Part model, mm, in its own coordinate system. A direction names the side the tool comes from. Give positions to 0.01 mm unless a question says otherwise; leave off trailing zeros. Order: outer loops, then holes, each group sorted by start corner. A loop starts at its lowest first (then second) coordinate and runs counter-clockwise, first axis right, second up. Notation, with made-up numbers: (-23.5, 15.5) - (15.5, 15.5) arc R25 ccw to (15.5, 32.5) - close; hole circle Ø2 at (-4.5, 84.25). An arc over 180 degrees is marked (long way). One line per item, written item: value.
```python
from build123d import *

# Parameters (mm, degrees)
F0_R     = 11.1125
F0_R_2   = 6.35
F1_DEPTH = 250.825
F2_DEPTH = 53.975
F3_SIZE2 = 1.5875
F3_SIZE  = 1.5875


with BuildPart() as f1:
    # F0 (on Top) → F1 (new body)
    with BuildSketch(Plane.XY):
        Circle(F0_R)
        Circle(F0_R_2, mode=Mode.SUBTRACT)
        Circle(F0_R_2)
    extrude(amount=F1_DEPTH)

    # F0 (on Top) → F2 (join)
    with BuildSketch(Plane.XY):
        Circle(F0_R_2)
    extrude(amount=-F2_DEPTH)

    # F3
    f3_edges = [f1.edges().sort_by_distance(p)[0] for p in [
        (-11.1125, 0, 250.825),
        (-6.35, 0, -53.975),
    ]]
    chamfer(f3_edges, length=F3_SIZE, length2=F3_SIZE2)


solid = f1.part
```
1) Wall check: line 1 along Z through (x, y) = (5.75, -4.75) (3 decimals); line 2 along Y through (x, z) = (-0.5, 16); line 3 along Y through (x, z) = (8.75, 136). Give the ranges that are in metal, low to high. Write a range as [from, to].
Answer:
line 1: z = [0, 250.825]
line 2: y = [-11.1, 11.1]
line 3: y = [-6.85, 6.85]
2) Slice it at C-C on z = 80.5. Write the cut outline in (x, y) (1 decimal), then the cut area to 3 significant figures.
Answer:
outline: circle Ø22.2 at (0, 0)
area: 388 mm2
3) Which spindle directions (+Z, -Z, +X, -X, +Y, -Y) get a long thin tool onto all of the face, cutting with end or side? Do faces 1 (the face through (-1.38, -6.2, -25.83)), 2 (the face through (0, 0, 250.825)). Say none if no direction does.
Answer:
face 1: -Z
face 2: +Z, +X, -X, +Y, -Y
4) Drop flat-ended pins along their axis: P1, Ø2, axis at x = 7.5, y = 0.5, coming from the -Z side; P2, Ø12, axis at x = 5.5, y = 0.5, coming from the -Z side (3 decimals); P3, Ø3, axis at y = 8.5, z = 47.5, coming from the +X side; P4, Ø6, axis at x = 4, z = 189.5, coming from the -Y side. Give the stop position or say it passes through.
Answer:
P1: stops at z = 0
P2: stops at z = -53.975
P3: stops at x = 8.63
P4: stops at y = -11.07
